from build123d import *

# Parameters (mm, degrees)
SKETCH1_R               = 10
BOSS_EXTRUDE2_DEPTH     = 5
BOSS_EXTRUDE3_DEPTH     = 55
BOSS_EXTRUDE4_START     = 50
SKETCH1_4_R             = 10
BOSS_EXTRUDE4_DEPTH     = 5
CUT_EXTRUDE2_DEPTH      = 1030.927549364
CUT_EXTRUDE2_DEPTH_BACK = 1030.927549364
CUT_EXTRUDE4_DEPTH      = 1029.839273162
CUT_EXTRUDE4_DEPTH_BACK = 1029.839273162
SKETCH5_W               = 8.968511721
SKETCH5_H               = 45
BOSS_EXTRUDE5_DEPTH     = 319


with BuildPart() as part:
    # Sketch1 → Boss-Extrude2 (new body)
    with BuildSketch(Plane.XY):
        with BuildLine():
            Line((27.006290467, 987.419065417), (27, 1000))
            ThreePointArc((27, 1000), (11.625043938, 1024.369209126), (-16.989507662, 1020.984676061))
            ThreePointArc((-16.989507662, 1020.984676061), (-24.369209126, 1011.625043938), (-27, 1000))
            Line((-27, 1000), (-27.006290467, 987.419065417))
            Line((-27.006290467, 987.419065417), (-17.006290467, 987.419065417))
            Line((-17.006290467, 987.419065417), (-17.318511721, 362.976557611))
            Line((-17.318511721, 362.976557611), (-27.318511721, 362.976557611))
            Line((-27.318511721, 362.976557611), (-27.5, 0))
            ThreePointArc((-27.5, 0), (0, -27.5), (27.5, 0))
            Line((27.5, 0), (27.318511721, 362.976557611))
            Line((27.318511721, 362.976557611), (17.318511721, 362.976557611))
            Line((17.318511721, 362.976557611), (17.006290467, 987.419065417))
            Line((17.006290467, 987.419065417), (27.006290467, 987.419065417))
        make_face()
        Circle(SKETCH1_R, mode=Mode.SUBTRACT)
        with Locations((0, 1000)):
            Circle(SKETCH1_R, mode=Mode.SUBTRACT)
    extrude(amount=BOSS_EXTRUDE2_DEPTH)

    # Sketch1<3> → Boss-Extrude3 (add)
    with BuildSketch(Plane.XY):
        Polygon((27.318511721, 362.976557611), (27.006290467, 987.419065417), (17.006290467, 987.419065417), (17.318511721, 362.976557611), align=None)
        Polygon((-17.006290467, 987.419065417), (-27.006290467, 987.419065417), (-27.318511721, 362.976557611), (-17.318511721, 362.976557611), align=None)
    extrude(amount=BOSS_EXTRUDE3_DEPTH)

    # Sketch1<4> → Boss-Extrude4 (add)
    with BuildSketch(Plane.XY.offset(BOSS_EXTRUDE4_START)):
        with BuildLine():
            Line((27, 1000), (27.5, 0))
            ThreePointArc((27.5, 0), (0, -27.5), (-27.5, 0))
            Line((-27.5, 0), (-27, 1000))
            ThreePointArc((-27, 1000), (0, 1027), (27, 1000))
        make_face()
        Circle(SKETCH1_4_R, mode=Mode.SUBTRACT)
        with Locations((0, 1000)):
            Circle(SKETCH1_4_R, mode=Mode.SUBTRACT)
    extrude(amount=BOSS_EXTRUDE4_DEPTH)

    # Sketch3 → Cut-Extrude2 (cut, two sides: drawn at the far end of the back side and taken through both)
    with BuildSketch(Plane(origin=(27.499993125, 0.013749997, 0), x_dir=(0, 0, -1), z_dir=(0.9999998750000234, 0.0004999999375000122, 0)).offset(-CUT_EXTRUDE2_DEPTH_BACK)):
        Polygon((-9.15125207, 508.572247167), (-9.15125207, 612.557963539), (-41.657857257, 612.557963539), align=None)
        Polygon((-9.15125207, 273.788247167), (-9.15125207, 481.759679911), (-41.657857257, 377.773963539), align=None)
        Polygon((-13.342142743, 495.165963539), (-45.84874793, 599.151679911), (-45.84874793, 391.180247167), align=None)
    extrude(amount=CUT_EXTRUDE2_DEPTH + CUT_EXTRUDE2_DEPTH_BACK, mode=Mode.SUBTRACT)

    # Sketch4 → Cut-Extrude4 (cut, two sides: drawn at the far end of the back side and taken through both)
    with BuildSketch(Plane.XY.offset(55).offset(-CUT_EXTRUDE4_DEPTH_BACK)):
        Polygon((14.164977662, 264.312281668), (-18.35, 369.999248569), (-18.35, 158.625314767), align=None)
        Polygon((18.35, 277.915314767), (18.35, 383.602281668), (-14.164977662, 383.602281668), align=None)
        Polygon((18.35, 39.335314767), (18.35, 250.709248569), (-14.164977662, 145.022281668), align=None)
        Polygon((14.164977662, 502.892281668), (-18.35, 608.579248569), (-18.35, 397.205314767), align=None)
        Polygon((18.35, 383.602281668), (18.35, 489.289248569), (-14.164977662, 383.602281668), align=None)
        Polygon((18.35, 516.495314767), (18.35, 622.182281668), (-14.164977662, 622.182281668), align=None)
        Polygon((14.164712586, 25.733143274), (-18.35, 131.419248569), (-18.35, 25.733143274), align=None)
    extrude(amount=CUT_EXTRUDE4_DEPTH + CUT_EXTRUDE4_DEPTH_BACK, mode=Mode.SUBTRACT)

    # Sketch5 → Boss-Extrude5 (add)
    with BuildSketch(Plane.XZ.offset(-362.976557611)):
        with Locations((-22.834255861, 27.5)):
            Rectangle(SKETCH5_W, SKETCH5_H)
        with Locations((22.834255861, 27.5)):
            Rectangle(SKETCH5_W, SKETCH5_H)
    extrude(amount=BOSS_EXTRUDE5_DEPTH)


solid = part.part
For this review, take the finished solid that the model builds, in its own axes (mm). A direction names the side the tool comes from. Round coordinates to 2 decimals unless told otherwise and drop trailing zeros. Order: outer loops, then holes, each group sorted by start corner. A loop starts at its lowest first (then second) coordinate and runs counter-clockwise, first axis right, second up. Notation, with made-up numbers: (74, 17) -> (125, 17) arc R17 ccw to (125, 43) -> close; hole circle Ø10 at (8.5, -38.5). An arc over 180 degrees is marked (long way). Write item = value, one per line. Start each with the question number.
1) To check wall thickness, follow line 1 (X direction, y = 1000, z = 3); line 2 (Z direction, x = 5.5, y = 835); line 3 (X direction, y = 585, z = 37.5). State the ranges of each line that lie inside material, in increasing order. Write a range as from..to.
2) The part is to be moulded in two halves that separate along Y. For faces 3 (the face through (-0.605, -27.493, 2.465)), 4 (the face through (-2.17, -9.76, 2.46)), 5 (the face through (-0.594, 1026.993, 52.465)), say which applies: +Y half, -Y half, draft (parallel to the pull), parting line (faces both ways), or undercut.
3) Insertion check: pin 1 (6 mm diameter, centred on y = 479, z = 11.5, fed in from +X); pin 2 (12 mm diameter, centred on y = 171.5, z = 22.5, fed in from -X); pin 3 (5.5 mm diameter, centred on x = 0, z = 52, fed in from +Y). Each pin has a flat end and moves straight along its axis. Give the tip position at first contact, or say it passes through.
4) Take a section at A-A on y = 208. State the section outline as (x, z) points.
5) Take a section at B-B on y = 945. State the section outline as (x, z) points.
6) Tool access review of faces 1 (the face through (0, 624, 55)), 2 (the face through (18, 622.182, 23)): name each direction out of +Z, -Z, +X, -X, +Y, -Y from which nothing blocks a thin tool from reaching the whole face with its end or side.
7) Take a section at C-C on x = 0. Count the separate pieces of the cut face and the enclosed holes in it, plus the area to 3 significant figures.
8) Take a section at D-D on y = 704.5. State the section outline as (x, z) points, plus the area to 3 significant figures.
Verdict:
q1.line_1 = -27..-10, 10..27
q1.line_2 = 0..5, 50..55
q1.line_3 = -27.21..-18.35, 18.35..27.21
q2.face_3 = -Y half
q2.face_4 = undercut
q2.face_5 = +Y half
q3.pin_1 = 27.26
q3.pin_2 = -27.32
q3.pin_3 = 1027
q4.outline = (-27.4, 0) -> (-18.35, 0) -> (-18.35, 55) -> (-27.4, 55) -> (-27.4, 50) -> (-27.32, 50) -> (-27.32, 5) -> (-27.4, 5) -> close; (-3.16, 0) -> (5.21, 0) -> (5.21, 5) -> (-3.16, 5) -> close; (-3.16, 50) -> (5.21, 50) -> (5.21, 55) -> (-3.16, 55) -> close; (18.35, 0) -> (27.4, 0) -> (27.4, 5) -> (27.32, 5) -> (27.32, 50) -> (27.4, 50) -> (27.4, 55) -> (18.35, 55) -> close
q5.outline = (-27.03, 0) -> (27.03, 0) -> (27.03, 55) -> (-27.03, 55) -> close; hole (-17.03, 5) -> (17.03, 5) -> (17.03, 50) -> (-17.03, 50) -> close
q6.face_1 = +Z, +X, -X, +Y, -Y
q6.face_2 = +Z, -Z
q7.separate_pieces = 18
q7.enclosed_holes = 0
q7.area = 5,540 mm2
q8.outline = (-27.15, 0) -> (27.15, 0) -> (27.15, 55) -> (-27.15, 55) -> close; hole (-17.15, 5) -> (17.15, 5) -> (17.15, 50) -> (-17.15, 50) -> close
q8.area = 1,440 mm2
